```python
from build123d import *

# Parameters (mm, degrees)
SKETCH1_W                           = 9
SKETCH1_H                           = 12
EXTRUDE1_DEPTH                      = 3.175
SKETCH2_W                           = 7
SKETCH2_H                           = 7
EXTRUDE2_DEPTH                      = 3.5
F_0_80_TAPPED_HOLE1_D               = 1.19126
F_0_80_TAPPED_HOLE1_DEPTH           = 4
F_0_80_TAPPED_HOLE1_TIP             = 0.357890611
F_3_32_0_09375_DIAMETER_HOLE1_D     = 2.38125
F_3_32_0_09375_DIAMETER_HOLE1_DEPTH = 10
F_3_32_0_09375_DIAMETER_HOLE1_TIP   = 0.715399675
FILLET7_R                           = 1


with BuildPart() as part:
    # Sketch1 → Extrude1 (new body)
    with BuildSketch(Plane(origin=(0, 0, 0), x_dir=(1, 0, 0), z_dir=(0, 1, 0))):
        Rectangle(SKETCH1_W, SKETCH1_H)
    extrude(amount=EXTRUDE1_DEPTH)

    # Sketch2 → Extrude2 (cut)
    with BuildSketch(Plane(origin=(0, 3.175, 0), x_dir=(1, 0, 0), z_dir=(0, 1, 0))):
        with Locations((0, -1.5)):
            Rectangle(SKETCH2_W, SKETCH2_H)
    extrude(amount=-EXTRUDE2_DEPTH, mode=Mode.SUBTRACT)

    # #0-80 Tapped Hole1
    with Locations(Plane(origin=(0, 3.175, -4), x_dir=(0, 0, 1), z_dir=(0, 1, 0))):
        with Locations((0, 0)):
            Hole(F_0_80_TAPPED_HOLE1_D / 2, depth=F_0_80_TAPPED_HOLE1_DEPTH)
            with Locations((0, 0, -(F_0_80_TAPPED_HOLE1_DEPTH + F_0_80_TAPPED_HOLE1_TIP / 2))):  # 118° drill point
                Cone(0, F_0_80_TAPPED_HOLE1_D / 2, F_0_80_TAPPED_HOLE1_TIP, mode=Mode.SUBTRACT)

    # 3/32 (0.09375) Diameter Hole1
    with Locations(Plane(origin=(-2.5, 3.175, -4), x_dir=(0, 0, 1), z_dir=(0, 1, 0))):
        with Locations((0, 0), (0, 5)):
            Hole(F_3_32_0_09375_DIAMETER_HOLE1_D / 2, depth=F_3_32_0_09375_DIAMETER_HOLE1_DEPTH)
            with Locations((0, 0, -(F_3_32_0_09375_DIAMETER_HOLE1_DEPTH + F_3_32_0_09375_DIAMETER_HOLE1_TIP / 2))):  # 118° drill point
                Cone(0, F_3_32_0_09375_DIAMETER_HOLE1_D / 2, F_3_32_0_09375_DIAMETER_HOLE1_TIP, mode=Mode.SUBTRACT)

    # Fillet7
    fillet7_edges = [part.edges().sort_by_distance(p)[0] for p in [
        (-3.5, 1.5875, 5),
        (-3.5, 1.5875, -2),
        (3.5, 1.5875, -2),
        (3.5, 1.5875, 5),
        (-4.5, 1.5875, -6),
        (4.5, 1.5875, -6),
        (4.5, 1.5875, 6),
        (-4.5, 1.5875, 6),
    ]]
    fillet(fillet7_edges, radius=FILLET7_R)


solid = part.part
```
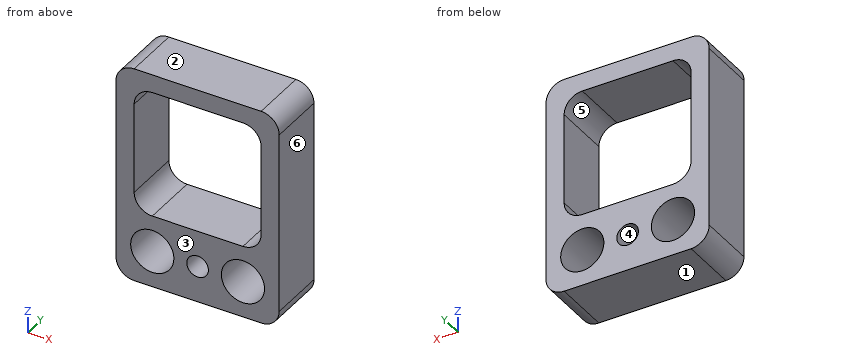
Geometry: final body of the model. Coordinates: model frame, mm. Face numbers are marked on the shaded views. A direction names the side the tool comes from. Coordinates: 2 decimals unless noted, no trailing zeros. Order: outer loops, then holes, each group sorted by start corner. A loop starts at its lowest first (then second) coordinate and runs counter-clockwise, first axis right, second up. Notation, with made-up numbers: (32.25, 25.25) -> (55.25, 25.25) arc R12 cw to (55.25, 44.25) -> close; hole circle Ø1 at (17.25, 31). An arc over 180 degrees is marked (long way). Write each question's results on one line, items separated by ' | '. Start each with the question number.
1) Cut plane B-B, the plane y = 0.9. Output: boundary loops of the cut face in (x, z), and give its area (3 significant figures).
2) Cut plane A-A, the plane z = -4. Output: boundary loops of the cut face in (x, y) (3 decimals), and give its area (3 significant figures).
3) Material intervals for line 1 along X through (y, z) = (1.4, -4); line 2 along Z through (x, y) = (0.75, 2.05); line 3 along X through (y, z) = (0.8, -0.25), sorted ascending.
4) Cut plane D-D, the plane x = -1. Output: boundary loops of the cut face in (y, z) (3 decimals).
5) Mould query, pull axis Z, two halves, no side actions, for the marked faces 1, 2, 3 and 4. Classes: released by +Z, released by -Z, zero draft, split by the parting line, or undercut.
6) Cut plane C-C, the plane z = 2. Output: boundary loops of the cut face in (x, y) (3 decimals).
7) First-contact query: pin 1 (1.4 mm diameter, centred on x = 2.5, z = -4, fed in from +Y). Flat tip, straight axial feed; report the tip coordinate or a pass-through.
8) Set-up query: the marked faces 5 and 6. Return all of +Z, -Z, +X, -X, +Y, -Y with unobstructed straight access to the full face (end or side cutting, diameter ignored); none if empty.
Checks:
1) outline: (-4.5, -5) arc R1 ccw to (-3.5, -6) -> (3.5, -6) arc R1 ccw to (4.5, -5) -> (4.5, 5) arc R1 ccw to (3.5, 6) -> (-3.5, 6) arc R1 ccw to (-4.5, 5) -> close; hole circle Ø2.38 at (-2.5, -4); hole (-3.5, -1) arc R1 ccw to (-2.5, -2) -> (2.5, -2) arc R1 ccw to (3.5, -1) -> (3.5, 4) arc R1 ccw to (2.5, 5) -> (-2.5, 5) arc R1 ccw to (-3.5, 4) -> close; hole circle Ø1.19 at (0, -4); hole circle Ø2.38 at (2.5, -4) | area: 49.0 mm^2
2) outline: (-4.5, 0) -> (-3.691, 0) -> (-3.691, 3.175) -> (-4.5, 3.175) -> close; (-1.309, 0) -> (-0.596, 0) -> (-0.596, 3.175) -> (-1.309, 3.175) -> close; (0.596, 0) -> (1.309, 0) -> (1.309, 3.175) -> (0.596, 3.175) -> close; (3.691, 0) -> (4.5, 0) -> (4.5, 3.175) -> (3.691, 3.175) -> close | area: 9.67 mm^2
3) line 1: -4.5 to -3.69, -1.31 to -0.6, 0.6 to 1.31, 3.69 to 4.5 | line 2: -6 to -2, 5 to 6 | line 3: -4.5 to -3.5, 3.5 to 4.5
4) outline: (0, -6) -> (3.175, -6) -> (3.175, -2) -> (0, -2) -> close; (0, 5) -> (3.175, 5) -> (3.175, 6) -> (0, 6) -> close
5) face 1: released by -Z | face 2: released by +Z | face 3: zero draft | face 4: undercut
6) outline: (-4.5, 0) -> (-3.5, 0) -> (-3.5, 3.175) -> (-4.5, 3.175) -> close; (3.5, 0) -> (4.5, 0) -> (4.5, 3.175) -> (3.5, 3.175) -> close
7) pin 1: through
8) face 5: +Y, -Y | face 6: +Z, -Z, +X, +Y, -Y
